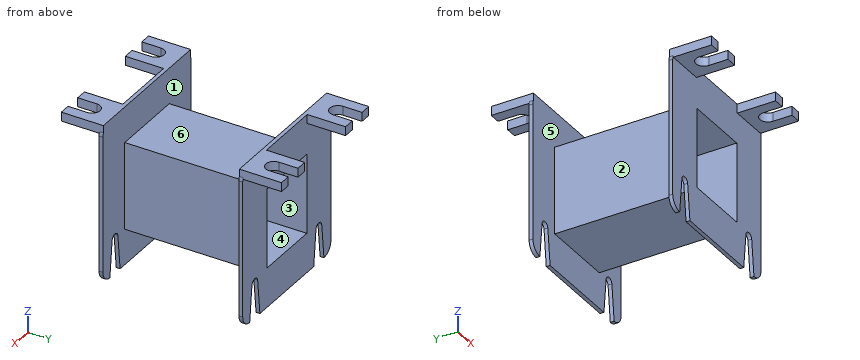
```python
from build123d import *

# Parameters (mm, degrees)
SKETCH1_W           = 17.2
SKETCH1_H           = 20.8
BOSS_EXTRUDE1_DEPTH = 1
SKETCH2_W           = 19.2
SKETCH2_H           = 22.8
SKETCH2_W_2         = 17.2
SKETCH2_H_2         = 20.8
BOSS_EXTRUDE2_DEPTH = 35.5
SKETCH3_W           = 17.2
SKETCH3_H           = 20.8
BOSS_EXTRUDE3_DEPTH = 1
CUT_EXTRUDE1_DEPTH  = 38.5
BOSS_EXTRUDE4_DEPTH = 11
SKETCH8_W           = 10
SKETCH8_H           = 2.35
BOSS_EXTRUDE5_DEPTH = 11
CUT_EXTRUDE2_DEPTH  = 42.5


with BuildPart() as part:
    # Sketch1 → Boss-Extrude1 (new body)
    with BuildSketch(Plane(origin=(0, 0, 0), x_dir=(1, 0, 0), z_dir=(0, 1, 0))):
        with BuildLine():
            Line((-16, -20.75), (16, -20.75))
            ThreePointArc((16, -20.75), (18.121320344, -19.871320344), (19, -17.75))
            Line((19, -17.75), (19, 17.75))
            ThreePointArc((19, 17.75), (18.121320344, 19.871320344), (16, 20.75))
            Line((16, 20.75), (-16, 20.75))
            ThreePointArc((-16, 20.75), (-18.121320344, 19.871320344), (-19, 17.75))
            Line((-19, 17.75), (-19, -17.75))
            ThreePointArc((-19, -17.75), (-18.121320344, -19.871320344), (-16, -20.75))
        make_face()
        Rectangle(SKETCH1_W, SKETCH1_H, mode=Mode.SUBTRACT)
    extrude(amount=BOSS_EXTRUDE1_DEPTH)

    # Sketch2 → Boss-Extrude2 (add)
    with BuildSketch(Plane(origin=(0, 1, 0), x_dir=(1, 0, 0), z_dir=(0, 1, 0))):
        Rectangle(SKETCH2_W, SKETCH2_H)
        Rectangle(SKETCH2_W_2, SKETCH2_H_2, mode=Mode.SUBTRACT)
    extrude(amount=BOSS_EXTRUDE2_DEPTH)

    # Sketch3 → Boss-Extrude3 (add)
    with BuildSketch(Plane(origin=(0, 36.5, 0), x_dir=(1, 0, 0), z_dir=(0, 1, 0))):
        with BuildLine():
            Line((-16, -20.75), (16, -20.75))
            ThreePointArc((16, -20.75), (18.121320344, -19.871320344), (19, -17.75))
            Line((19, -17.75), (19, 17.75))
            ThreePointArc((19, 17.75), (18.121320344, 19.871320344), (16, 20.75))
            Line((16, 20.75), (-16, 20.75))
            ThreePointArc((-16, 20.75), (-18.121320344, 19.871320344), (-19, 17.75))
            Line((-19, 17.75), (-19, -17.75))
            ThreePointArc((-19, -17.75), (-18.121320344, -19.871320344), (-16, -20.75))
        make_face()
        Rectangle(SKETCH3_W, SKETCH3_H, mode=Mode.SUBTRACT)
    extrude(amount=BOSS_EXTRUDE3_DEPTH)

    # Sketch4 → Cut-Extrude1 (cut, through all)
    with BuildSketch(Plane(origin=(0, 37.5, 0), x_dir=(-1, 0, 0), z_dir=(0, 1, 0))):
        with BuildLine():
            Line((11.6, -20.75), (12.572602238, -11.413367935))
            ThreePointArc((12.572602238, -11.413367935), (13.8, -10.4), (15.027397762, -11.413367935))
            Line((15.027397762, -11.413367935), (16, -20.75))
            Line((16, -20.75), (11.6, -20.75))
        make_face()
        with BuildLine():
            Line((-11.6, -20.75), (-12.572602238, -11.413367935))
            ThreePointArc((-12.572602238, -11.413367935), (-13.8, -10.4), (-15.027397762, -11.413367935))
            Line((-15.027397762, -11.413367935), (-16, -20.75))
            Line((-16, -20.75), (-11.6, -20.75))
        make_face()
    extrude(amount=-CUT_EXTRUDE1_DEPTH, mode=Mode.SUBTRACT)

    # Sketch6 → Boss-Extrude4 (add)
    with BuildSketch(Plane.XZ.offset(-36.5)):
        Polygon((-13.8, 20.75), (-18.8, 20.75), (-18.8, 18.4), (-8.8, 18.4), (-8.8, 20.75), align=None)
        Polygon((8.8, 18.4), (8.8, 20.75), (13.8, 20.75), (18.8, 20.75), (18.8, 18.4), align=None)
    extrude(amount=-BOSS_EXTRUDE4_DEPTH)

    # Sketch8 → Boss-Extrude5 (add)
    with BuildSketch(Plane(origin=(0, 1, 0), x_dir=(1, 0, 0), z_dir=(0, 1, 0))):
        with Locations((-13.8, -19.575)):
            Rectangle(SKETCH8_W, SKETCH8_H)
        with Locations((13.8, -19.575)):
            Rectangle(SKETCH8_W, SKETCH8_H)
    extrude(amount=-BOSS_EXTRUDE5_DEPTH)

    # Sketch9 → Cut-Extrude2 (cut, through all)
    with BuildSketch(Plane.XY.offset(20.75)):
        with BuildLine():
            Line((-15.9, -4.996046188), (-15.9, -10))
            Line((-15.9, -10), (-11.7, -10))
            Line((-11.7, -10), (-11.7, -4.996046188))
            ThreePointArc((-11.7, -4.996046188), (-13.8, -2.896046188), (-15.9, -4.996046188))
        make_face()
        with BuildLine():
            Line((15.9, -10), (11.7, -10))
            Line((11.7, -10), (11.7, -4.996046188))
            ThreePointArc((11.7, -4.996046188), (13.8, -2.896046188), (15.9, -4.996046188))
            Line((15.9, -4.996046188), (15.9, -10))
        make_face()
        with BuildLine():
            Line((15.9, 47.5), (11.7, 47.5))
            Line((11.7, 47.5), (11.7, 42.496046188))
            ThreePointArc((11.7, 42.496046188), (13.8, 40.396046188), (15.9, 42.496046188))
            Line((15.9, 42.496046188), (15.9, 47.5))
        make_face()
        with BuildLine():
            Line((-15.9, 47.5), (-11.7, 47.5))
            Line((-11.7, 47.5), (-11.7, 42.496046188))
            ThreePointArc((-11.7, 42.496046188), (-13.8, 40.396046188), (-15.9, 42.496046188))
            Line((-15.9, 42.496046188), (-15.9, 47.5))
        make_face()
    extrude(amount=-CUT_EXTRUDE2_DEPTH, mode=Mode.SUBTRACT)


solid = part.part
```
Input: part model. Units: mm. Frame: model coordinates. Face numbers are marked on the shaded views. A direction names the side the tool comes from. Coordinates: 2 decimals unless noted, no trailing zeros. Write each loop counter-clockwise with the first axis right and the second up, starting at its lowest first coordinate (ties: lowest second). Pieces come first, ordered by that corner, then holes. Notation, with made-up numbers: M -37.5,36.5 L -1.5,36.5 A15 ccw -1.5,60.5 Z; hole C 88,10.5 d5. An arc over 180 degrees is marked long. Use one line per item in the form item = value.
Q1. Section D-D (z = -15.5). Return loops of the section in (x, y), plus the area to 3 significant figures.
Answer below:
outline = M -19,0 L -15.45,0 L -15.45,1 L -19,1 Z; M -19,36.5 L -15.45,36.5 L -15.45,37.5 L -19,37.5 Z; M -12.15,0 L 12.15,0 L 12.15,1 L -12.15,1 Z; M -12.15,36.5 L 12.15,36.5 L 12.15,37.5 L -12.15,37.5 Z; M 15.45,0 L 19,0 L 19,1 L 15.45,1 Z; M 15.45,36.5 L 19,36.5 L 19,37.5 L 15.45,37.5 Z
area = 62.8 mm²
Q2. Section B-B (x = 10.5). Return loops of the section in (y, z).
Answer below:
outline = M -10,18.4 L 0,18.4 L 0,-20.75 L 1,-20.75 L 1,20.75 L -10,20.75 Z; M 36.5,-20.75 L 37.5,-20.75 L 37.5,18.4 L 47.5,18.4 L 47.5,20.75 L 36.5,20.75 Z
Q3. Section A-A (z = 0.5). Return loops of the section in (x, y).
Answer below:
outline = M -19,0 L -8.6,0 L -8.6,37.5 L -19,37.5 L -19,36.5 L -9.6,36.5 L -9.6,1 L -19,1 Z; M 8.6,0 L 19,0 L 19,1 L 9.6,1 L 9.6,36.5 L 19,36.5 L 19,37.5 L 8.6,37.5 Z
Q4. Material intervals for probe 1 along X at (y, z) = (-2, 19); probe 2 along Z at (x, y) = (5, 30); probe 3 along Y at (x, z) = (10.5, 18), sorted ascending. Write a range as from..to.
Answer below:
probe_1 = -18.8..-8.8, 8.8..18.8
probe_2 = -11.4..-10.4, 10.4..11.4
probe_3 = 0..1, 36.5..37.5
Q5. First-contact query: pin 1 (8 mm diameter, centred on x = -14.5, y = 43.5, fed in from -Z); pin 2 (19 mm diameter, centred on x = -1, y = 9.5, fed in from -Z); pin 3 (1.9 mm diameter, centred on y = 45, z = 19, fed in from -X); pin 4 (2 mm diameter, centred on x = -7.5, z = 13, fed in from +Y). Flat tips, straight axial feed; report the tip coordinate or a pass-through.
Answer below:
pin_1 = 18.4
pin_2 = -20.75
pin_3 = -18.8
pin_4 = 37.5
Q6. Draft query along Z for the marked faces 4, 5 and 6. Return one class per face: released by +Z, released by -Z, zero draft, split by the parting line, or undercut.
Answer below:
face_4 = undercut
face_5 = zero draft
face_6 = released by +Z
Q7. Set-up query: the marked faces 1, 2 and 3. Return all of +Z, -Z, +X, -X, +Y, -Y with unobstructed straight access to the full face (end or side cutting, diameter ignored); none if empty.
Answer below:
face_1 = none
face_2 = +Z, -Z, -X
face_3 = +Y, -Y
Q8. Section C-C (y = 34). Return loops of the section in (x, z), plus the area to 3 significant figures.
Answer below:
outline = M -9.6,-11.4 L 9.6,-11.4 L 9.6,11.4 L -9.6,11.4 Z; hole M -8.6,-10.4 L 8.6,-10.4 L 8.6,10.4 L -8.6,10.4 Z
area = 80.0 mm²
